from build123d import *

# Parameters (mm, degrees)
SKETCH1_W               = 50
SKETCH1_H               = 34.11
BOSS_EXTRUDE1_DEPTH     = 20
SKETCH2_R               = 3
BOSS_EXTRUDE2_DEPTH     = 9.5
LPATTERN1_COUNT         = 3
LPATTERN1_PITCH         = 20.25
MIRROR1_COPY_1_SKETCH_R = 3
MIRROR1_COPY_1_DEPTH    = 9.5
MIRROR1_COPY_2_SKETCH_R = 3
MIRROR1_COPY_2_DEPTH    = 9.5
SKETCH3_R               = 8
SKETCH3_W               = 3
SKETCH3_H               = 30
CUT_EXTRUDE1_DEPTH      = 10
SKETCH4_W               = 42
SKETCH4_H               = 22.11
CUT_EXTRUDE2_DEPTH      = 3
FILLET1_R               = 6
FILLET2_R               = 6
BOSS_EXTRUDE3_START     = 20
SKETCH5_W               = 25
SKETCH5_H               = 22.11
SKETCH5_R               = 8
BOSS_EXTRUDE3_DEPTH     = 20


with BuildPart() as part:
    # Sketch1 → Boss-Extrude1 (new body)
    with BuildSketch(Plane(origin=(0, 0, 0), x_dir=(0, 0, -1), z_dir=(1, 0, 0))):
        with Locations((25, 17.055)):
            Rectangle(SKETCH1_W, SKETCH1_H)
    extrude(amount=BOSS_EXTRUDE1_DEPTH)

    # Sketch2 → Boss-Extrude2 (add)
    with BuildSketch(Plane.XY):
        with BuildLine():
            Line((20, 34.11), (25, 34.11))
            ThreePointArc((25, 34.11), (30, 39.11), (25, 44.11))
            Line((25, 44.11), (18, 44.11))
            Line((18, 44.11), (8, 34.11))
            Line((8, 34.11), (20, 34.11))
        make_face()
        with Locations((25, 39.11)):
            Circle(SKETCH2_R, mode=Mode.SUBTRACT)
    boss_extrude2 = extrude(amount=-BOSS_EXTRUDE2_DEPTH)

    # LPattern1: Boss-Extrude2 ×3
    with Locations(*[(0, 0, -i * LPATTERN1_PITCH) for i in range(1, LPATTERN1_COUNT)]):
        add(boss_extrude2)

    # Mirror1: Boss-Extrude2 across plane
    add(boss_extrude2.mirror(Plane.ZX.offset(17.055)))

    # Mirror1 copy 1 sketch → Mirror1 copy 1 (add)
    with BuildSketch(Plane(origin=(0, 34.11, -20.25), x_dir=(1, 0, 0), z_dir=(0, 0, 1))):
        with BuildLine():
            Line((20, -34.11), (25, -34.11))
            ThreePointArc((25, -34.11), (30, -39.11), (25, -44.11))
            Line((25, -44.11), (18, -44.11))
            Line((18, -44.11), (8, -34.11))
            Line((8, -34.11), (20, -34.11))
        make_face()
        with Locations((25, -39.11)):
            Circle(MIRROR1_COPY_1_SKETCH_R, mode=Mode.SUBTRACT)
    extrude(amount=-MIRROR1_COPY_1_DEPTH)

    # Mirror1 copy 2 sketch → Mirror1 copy 2 (add)
    with BuildSketch(Plane(origin=(0, 34.11, -40.5), x_dir=(1, 0, 0), z_dir=(0, 0, 1))):
        with BuildLine():
            Line((20, -34.11), (25, -34.11))
            ThreePointArc((25, -34.11), (30, -39.11), (25, -44.11))
            Line((25, -44.11), (18, -44.11))
            Line((18, -44.11), (8, -34.11))
            Line((8, -34.11), (20, -34.11))
        make_face()
        with Locations((25, -39.11)):
            Circle(MIRROR1_COPY_2_SKETCH_R, mode=Mode.SUBTRACT)
    extrude(amount=-MIRROR1_COPY_2_DEPTH)

    # Sketch3 → Cut-Extrude1 (cut)
    with BuildSketch(Plane.ZY):
        with Locations((-25, 17.055)):
            Circle(SKETCH3_R)
        with Locations((-39, 17.055)):
            Rectangle(SKETCH3_W, SKETCH3_H)
        with Locations((-11, 17.055)):
            Rectangle(SKETCH3_W, SKETCH3_H)
    extrude(amount=-CUT_EXTRUDE1_DEPTH, mode=Mode.SUBTRACT)

    # Sketch4 → Cut-Extrude2 (cut)
    with BuildSketch(Plane(origin=(0, 0, 0), x_dir=(0, 0, -1), z_dir=(1, 0, 0))):
        Polygon((50, 34.11), (0, 34.11), (0, 28.11), (0, 6), (0, 0), (50, 0), (50, 6), (50, 28.11), align=None)
        with Locations((25, 17.055)):
            Rectangle(SKETCH4_W, SKETCH4_H, mode=Mode.SUBTRACT)
    extrude(amount=CUT_EXTRUDE2_DEPTH, mode=Mode.SUBTRACT)

    # Fillet1
    # the kernel refuses this fillet: 6 mm, written as the material it adds along each edge
    with BuildSketch(Plane(origin=(20, 0, -25.613872125), x_dir=(0, 1, 0), z_dir=(0, 0, -1))) as fillet1_piece_1_section:
        with BuildLine():
            CenterArc((5.95445115, 6), FILLET1_R, 185.21590857, 84.78409143)
            Line((-0.020704023, 5.454545455), (-0.61821954, 5.4))
            ThreePointArc((-0.61821954, 5.4), (-0.6, 5), (-0.6, 0))
            Line((-0.6, 0), (0, -0.6))
            Line((0, -0.6), (5.95445115, -0.6))
            Line((5.95445115, -0.6), (5.95445115, 0))
        make_face()
    fillet1_piece_1 = extrude(amount=39.272255751, mode=Mode.PRIVATE)
    fillet1_piece_1 = split(fillet1_piece_1, bisect_by=Plane(origin=(21.495039794, 1.973310918, -29.75), z_dir=(0, 0, 1)), keep=Keep.TOP, mode=Mode.PRIVATE)
    add(fillet1_piece_1)
    with BuildSketch(Plane(origin=(20, 0, -40.5), x_dir=(0, 1, 0), z_dir=(0, 0, -1)), Plane(origin=(20, 0, -20.25), x_dir=(0, 1, 0), z_dir=(0, 0, -1)), Plane(origin=(20, 0, 0), x_dir=(0, 1, 0), z_dir=(0, 0, -1)), Plane(origin=(20, 34.11, -50), x_dir=(0, -1, 0), z_dir=(0, 0, 1)), Plane(origin=(20, 34.11, -29.75), x_dir=(0, -1, 0), z_dir=(0, 0, 1)), Plane(origin=(20, 34.11, -9.5), x_dir=(0, -1, 0), z_dir=(0, 0, 1))) as fillet1_piece_2:
        with BuildLine():
            CenterArc((5.95445115, 6), FILLET1_R, 185.21590857, 84.78409143)
            Line((-0.020704023, 5.454545455), (-0.61821954, 5.4))
            ThreePointArc((-0.61821954, 5.4), (-0.6, 5), (-0.6, 0))
            Line((-0.6, 0), (0, -0.6))
            Line((0, -0.6), (5.95445115, -0.6))
            Line((5.95445115, -0.6), (5.95445115, 0))
        make_face()
    extrude(amount=9.5)
    with BuildSketch(Plane(origin=(20, 0, -5.363872125), x_dir=(0, 1, 0), z_dir=(0, 0, -1))) as fillet1_piece_3_section:
        with BuildLine():
            CenterArc((5.95445115, 6), FILLET1_R, 185.21590857, 84.78409143)
            Line((-0.020704023, 5.454545455), (-0.61821954, 5.4))
            ThreePointArc((-0.61821954, 5.4), (-0.6, 5), (-0.6, 0))
            Line((-0.6, 0), (0, -0.6))
            Line((0, -0.6), (5.95445115, -0.6))
            Line((5.95445115, -0.6), (5.95445115, 0))
        make_face()
    fillet1_piece_3 = extrude(amount=39.272255751, mode=Mode.PRIVATE)
    fillet1_piece_3 = split(fillet1_piece_3, bisect_by=Plane(origin=(21.495039794, 1.973310918, -9.5), z_dir=(0, 0, 1)), keep=Keep.TOP, mode=Mode.PRIVATE)
    add(fillet1_piece_3)
    with BuildSketch(Plane(origin=(20, 0, -5.363872125), x_dir=(0, 1, 0), z_dir=(0, 0, -1))) as fillet1_piece_4_section:
        with BuildLine():
            CenterArc((5.95445115, 6), FILLET1_R, 185.21590857, 84.78409143)
            Line((-0.020704023, 5.454545455), (-0.61821954, 5.4))
            ThreePointArc((-0.61821954, 5.4), (-0.6, 5), (-0.6, 0))
            Line((-0.6, 0), (0, -0.6))
            Line((0, -0.6), (5.95445115, -0.6))
            Line((5.95445115, -0.6), (5.95445115, 0))
        make_face()
    fillet1_piece_4 = extrude(amount=39.272255751, mode=Mode.PRIVATE)
    fillet1_piece_4 = split(fillet1_piece_4, bisect_by=Plane(origin=(21.495039794, 1.973310918, -40.5), z_dir=(0, 0, -1)), keep=Keep.TOP, mode=Mode.PRIVATE)
    add(fillet1_piece_4)
    with BuildSketch(Plane(origin=(20, 0, 14.886127875), x_dir=(0, 1, 0), z_dir=(0, 0, -1))) as fillet1_piece_5_section:
        with BuildLine():
            CenterArc((5.95445115, 6), FILLET1_R, 185.21590857, 84.78409143)
            Line((-0.020704023, 5.454545455), (-0.61821954, 5.4))
            ThreePointArc((-0.61821954, 5.4), (-0.6, 5), (-0.6, 0))
            Line((-0.6, 0), (0, -0.6))
            Line((0, -0.6), (5.95445115, -0.6))
            Line((5.95445115, -0.6), (5.95445115, 0))
        make_face()
    fillet1_piece_5 = extrude(amount=39.272255751, mode=Mode.PRIVATE)
    fillet1_piece_5 = split(fillet1_piece_5, bisect_by=Plane(origin=(21.495039794, 1.973310918, -20.25), z_dir=(0, 0, -1)), keep=Keep.TOP, mode=Mode.PRIVATE)
    add(fillet1_piece_5)
    with BuildSketch(Plane(origin=(20, 34.11, -64.886127875), x_dir=(0, -1, 0), z_dir=(0, 0, 1))) as fillet1_piece_6_section:
        with BuildLine():
            CenterArc((5.95445115, 6), FILLET1_R, 185.21590857, 84.78409143)
            Line((-0.020704023, 5.454545455), (-0.61821954, 5.4))
            ThreePointArc((-0.61821954, 5.4), (-0.6, 5), (-0.6, 0))
            Line((-0.6, 0), (0, -0.6))
            Line((0, -0.6), (5.95445115, -0.6))
            Line((5.95445115, -0.6), (5.95445115, 0))
        make_face()
    fillet1_piece_6 = extrude(amount=39.272255751, mode=Mode.PRIVATE)
    fillet1_piece_6 = split(fillet1_piece_6, bisect_by=Plane(origin=(21.495039794, 32.136689082, -29.75), z_dir=(0, 0, 1)), keep=Keep.TOP, mode=Mode.PRIVATE)
    add(fillet1_piece_6)
    with BuildSketch(Plane(origin=(20, 34.11, -44.636127875), x_dir=(0, -1, 0), z_dir=(0, 0, 1))) as fillet1_piece_7_section:
        with BuildLine():
            CenterArc((5.95445115, 6), FILLET1_R, 185.21590857, 84.78409143)
            Line((-0.020704023, 5.454545455), (-0.61821954, 5.4))
            ThreePointArc((-0.61821954, 5.4), (-0.6, 5), (-0.6, 0))
            Line((-0.6, 0), (0, -0.6))
            Line((0, -0.6), (5.95445115, -0.6))
            Line((5.95445115, -0.6), (5.95445115, 0))
        make_face()
    fillet1_piece_7 = extrude(amount=39.272255751, mode=Mode.PRIVATE)
    fillet1_piece_7 = split(fillet1_piece_7, bisect_by=Plane(origin=(21.495039794, 32.136689082, -40.5), z_dir=(0, 0, -1)), keep=Keep.TOP, mode=Mode.PRIVATE)
    add(fillet1_piece_7)
    with BuildSketch(Plane(origin=(20, 34.11, -44.636127875), x_dir=(0, -1, 0), z_dir=(0, 0, 1))) as fillet1_piece_8_section:
        with BuildLine():
            CenterArc((5.95445115, 6), FILLET1_R, 185.21590857, 84.78409143)
            Line((-0.020704023, 5.454545455), (-0.61821954, 5.4))
            ThreePointArc((-0.61821954, 5.4), (-0.6, 5), (-0.6, 0))
            Line((-0.6, 0), (0, -0.6))
            Line((0, -0.6), (5.95445115, -0.6))
            Line((5.95445115, -0.6), (5.95445115, 0))
        make_face()
    fillet1_piece_8 = extrude(amount=39.272255751, mode=Mode.PRIVATE)
    fillet1_piece_8 = split(fillet1_piece_8, bisect_by=Plane(origin=(21.495039794, 32.136689082, -9.5), z_dir=(0, 0, 1)), keep=Keep.TOP, mode=Mode.PRIVATE)
    add(fillet1_piece_8)
    with BuildSketch(Plane(origin=(20, 34.11, -24.386127875), x_dir=(0, -1, 0), z_dir=(0, 0, 1))) as fillet1_piece_9_section:
        with BuildLine():
            CenterArc((5.95445115, 6), FILLET1_R, 185.21590857, 84.78409143)
            Line((-0.020704023, 5.454545455), (-0.61821954, 5.4))
            ThreePointArc((-0.61821954, 5.4), (-0.6, 5), (-0.6, 0))
            Line((-0.6, 0), (0, -0.6))
            Line((0, -0.6), (5.95445115, -0.6))
            Line((5.95445115, -0.6), (5.95445115, 0))
        make_face()
    fillet1_piece_9 = extrude(amount=39.272255751, mode=Mode.PRIVATE)
    fillet1_piece_9 = split(fillet1_piece_9, bisect_by=Plane(origin=(21.495039794, 32.136689082, -20.25), z_dir=(0, 0, -1)), keep=Keep.TOP, mode=Mode.PRIVATE)
    add(fillet1_piece_9)

    # Fillet2
    fillet2_edges = [part.edges().sort_by_distance(p)[0] for p in [
        (8, 0, -45.25),
        (8, 34.11, -4.75),
        (8, 34.11, -25),
        (8, 34.11, -45.25),
        (8, 0, -4.75),
        (8, 0, -25),
    ]]
    fillet(fillet2_edges, radius=FILLET2_R)

    # Sketch5 → Boss-Extrude3 (add)
    with BuildSketch(Plane.ZY.offset(BOSS_EXTRUDE3_START)):
        with Locations((-25, 17.055)):
            Rectangle(SKETCH5_W, SKETCH5_H)
        with Locations((-25, 17.055)):
            Circle(SKETCH5_R, mode=Mode.SUBTRACT)
    extrude(amount=-BOSS_EXTRUDE3_DEPTH)


solid = part.part
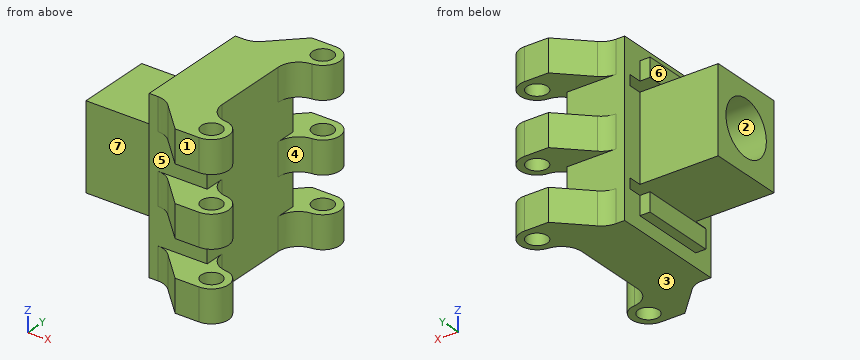
The listing builds one solid part. Answer for the finished solid, in the listing's coordinates (mm). Face numbers are marked on the shaded views. A direction names the side the tool comes from. Give positions to 0.01 mm unless a question says otherwise; leave off trailing zeros. Order: outer loops, then holes, each group sorted by start corner. A loop starts at its lowest first (then second) coordinate and runs counter-clockwise, first axis right, second up. Notation, with made-up numbers: (26, 41.25) - (77, 41.25) arc R21 ccw to (77, 65.25) - close; hole circle Ø7 at (78.5, -11.5). An arc over 180 degrees is marked (long way). One line per item, written item: value. Start each with the question number.
1) The mould has two halves that part along Z. Classify the marked faces 1, 2 and 3: released by +Z, released by -Z, zero draft, split by the parting line, or undercut.
2) A tool of negligible diameter and unlimited length cuts with its end or side. For the marked faces 4, 5, 6 and 7, from which of +Z, -Z, +X, -X, +Y, -Y can it reach the whole face along a straight path? Write none if from no direction.
3) A cutting plane is placed at A-A on y = -5. Give the vertices of the cut face in (x, z), then the cut area to 4 significant figures.
4) A cutting plane is placed at D-D on y = 26.5. Give the vertices of the cut face in (x, z).
5) Find the intervals of material crossed by L1, parallel to Z at x = 14, y = 35.5; L2, parallel to Y at x = 25, z = -7.25; L3, parallel to Z at x = 6, y = 15.5, in increasing order.
6) Given pin 1 Ø5 at (x, z) = (14, -29.5) entering from -Y; pin 2 Ø18.5 at (x, z) = (-12.5, -27.5) entering from -Y; pin 3 Ø7 at (x, y) = (25, 39.11) entering from +Z; pin 4 Ø10 at (y, z) = (22.5, -23.5) entering from +X, each flat-ended and moving along its own axis, determine where each tip first touches the part or whether it passes through.
7) A cutting plane is placed at B-B on z = -3. Give the vertices of the cut face in (x, y).
8) A cutting plane is placed at C-C on z = -10.5. Give the vertices of the cut face in (x, y) (3 decimals), then the cut area to 3 significant figures.
Answer sheet:
1. face 1: zero draft
1. face 2: undercut
1. face 3: released by -Z
2. face 4: +Z, -Z, +X
2. face 5: -X, -Y
2. face 6: +Z, -X, +Y, -Y
2. face 7: +Z, -Z, -X, -Y
3. outline: (13, -50) - (22, -50) - (22, -40.5) - (13, -40.5) - close; (13, -29.75) - (22, -29.75) - (22, -20.25) - (13, -20.25) - close; (13, -9.5) - (22, -9.5) - (22, 0) - (13, 0) - close; (28, -50) - (30, -50) - (30, -40.5) - (28, -40.5) - close; (28, -29.75) - (30, -29.75) - (30, -20.25) - (28, -20.25) - close; (28, -9.5) - (30, -9.5) - (30, 0) - (28, 0) - close
3. area: 313.5 mm2
4. outline: (-20, -37.5) - (10, -37.5) - (10, -40.5) - (0, -40.5) - (0, -46) - (3, -46) - (3, -50) - (20, -50) - (20, 0) - (3, 0) - (3, -4) - (0, -4) - (0, -9.5) - (10, -9.5) - (10, -12.5) - (-20, -12.5) - close
5. L1: z = -50 to -40.5, -29.75 to -20.25, -9.5 to 0
5. L2: y = -10 to -8, -2 to 0.04, 34.07 to 36.11, 42.11 to 44.11
5. L3: z = -50 to -40.5, -37.5 to -32.85, -17.15 to -12.5, -9.5 to 0
6. pin 1: stops at y = -8.5
6. pin 2: stops at y = 6
6. pin 3: stops at z = 0
6. pin 4: stops at x = 20
7. outline: (3, 0) - (5.51, 0) arc R6 cw to (9.76, -1.76) - (18, -10) - (25, -10) arc R5 ccw to (25.45, -0.02) arc R6 cw to (20, 5.95) - (20, 28.16) arc R6 cw to (25.45, 34.13) arc R5 ccw to (25, 44.11) - (18, 44.11) - (9.76, 35.87) arc R6 cw to (5.51, 34.11) - (3, 34.11) - close; hole circle Ø6 at (25, -5); hole circle Ø6 at (25, 39.11)
8. outline: (3, 0) - (20, 0) - (20, 34.11) - (3, 34.11) - (3, 32.055) - (10, 32.055) - (10, 2.055) - (3, 2.055) - close
8. area: 370 mm2
